```python
from build123d import *


with BuildPart() as part:
    # Sketch1 → Revolve1 (revolve)
    with BuildSketch(Plane.XY):
        with BuildLine():
            Line((0, 0.2921), (19.594743879, 0.2921))
            ThreePointArc((19.594743879, 0.2921), (22.024783674, 0.775464969), (24.084871939, 2.151971939))
            Line((24.084871939, 2.151971939), (29.890128061, 7.957228061))
            ThreePointArc((29.890128061, 7.957228061), (31.950216326, 9.333735031), (34.380256121, 9.8171))
            Line((34.380256121, 9.8171), (119.619043514, 9.8171))
            Line((119.619043514, 9.8171), (119.619043514, 16.9291))
            Line((119.619043514, 16.9291), (24.020959689, 37.2491))
            Line((24.020959689, 37.2491), (17.670959689, 37.2491))
            Line((17.670959689, 37.2491), (0, 6.6421))
            Line((0, 6.6421), (0, 0.2921))
        make_face()
    revolve(axis=Axis((0, 55.0291, 0), (1, 0, 0)))


solid = part.part
```
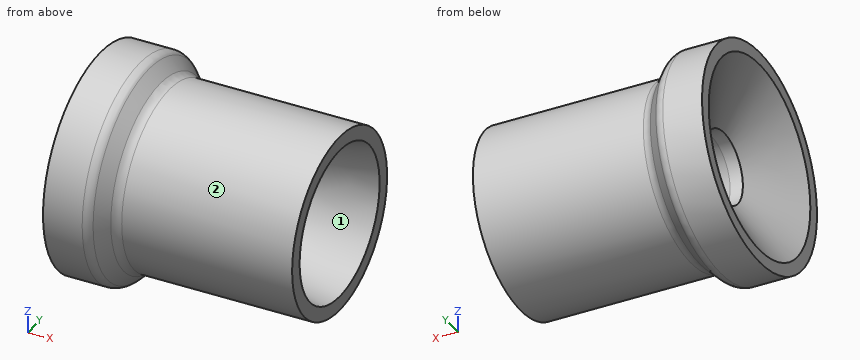
For this review, take the finished solid that the model builds, in its own axes (mm). Face numbers are marked on the shaded views. Give positions to 0.01 mm unless a question says otherwise; leave off trailing zeros. Write each loop counter-clockwise with the first axis right and the second up, starting at its lowest first coordinate (ties: lowest second). Pieces come first, ordered by that corner, then holes. Notation, with made-up numbers: M 12.5,46.25 L 30.5,46.25 A19 cw 30.5,66.25 Z; hole C 74.25,34.5 d11. An arc over 180 degrees is marked long. Answer as CSV lines item,"result".
1. Consider section A-A, the plane z = 0. Write out the cut boundary in (x, y), then the cut area to 3 significant figures.
Findings:
outline,"M 0,0.29 L 19.59,0.29 A6.35 ccw 24.08,2.15 L 29.89,7.96 A6.35 cw 34.38,9.82 L 119.62,9.82 L 119.62,16.93 L 24.02,37.25 L 17.67,37.25 L 0,6.64 Z; M 0,103.42 L 17.67,72.81 L 24.02,72.81 L 119.62,93.13 L 119.62,100.24 L 34.38,100.24 A6.35 cw 29.89,102.1 L 24.08,107.91 A6.35 ccw 19.59,109.77 L 0,109.77 Z"
area,"4,590 mm2"
2. Wall thickness on line 1 (Y direction, x = 20.5, z = 0); line 2 (Y direction, x = 21.25, z = 0); line 3 (Z direction, x = 111, y = 86): over which ranges is each line inside the solid? List them lowest first.
Findings:
line 1,"y = 0.36 to 37.25, 72.81 to 109.7"
line 2,"y = 0.51 to 37.25, 72.81 to 109.55"
line 3,"z = -32.94 to -18.87, 18.87 to 32.94"
3. Draft analysis for pull direction Z (two halves, no side actions). For the marked faces 1 and 2, state which applies: +Z half, -Z half, draft (parallel to the pull), parting line (faces both ways), or undercut.
Findings:
face 1,"undercut"
face 2,"parting line"
4. For pin 1 (1.5 mm diameter, centred on x = 24, z = -25, fed in from -Y); pin 2 (1 mm diameter, centred on x = 62, y = 41, fed in from +Z); pin 3 (2 mm diameter, centred on x = 81.5, z = -29.5, fed in from -Y); pin 4 (6 mm diameter, centred on y = 46, z = 36.5, fed in from +X), all flat-tipped, find the tip position at first contact; note any pin that passes through.
Findings:
pin 1,"stops at y = 7.52"
pin 2,"stops at z = 43.14"
pin 3,"stops at y = 19.93"
pin 4,"stops at x = 119.62"
5. Consider section C-C, the plane x = 75.5. Write out the cut boundary in (y, z).
Findings:
outline,"C 55.03,0 d90.42; hole C 55.03,0 d57.44"
6. Consider section B-B, the plane x = 59. Write out the cut boundary in (y, z).
Findings:
outline,"C 55.03,0 d90.42; hole C 55.03,0 d50.43"
